Source: three-view drawing plus pictorial views. Frame: mm from the lowest corner of the part. A direction names the side the tool comes from. Coordinates: 2 decimals unless noted, no trailing zeros. Order: outer loops, then holes, each group sorted by start corner. A loop starts at its lowest first (then second) coordinate and runs counter-clockwise, first axis right, second up. Notation, with made-up numbers: (-27, 2) -> (8, 2) arc R10 ccw to (8, 16) -> close; hole circle Ø1 at (23, 0.25). An arc over 180 degrees is marked (long way). Use one line per item in the form item = value. Start each with the question number.
1) Ray query, line 1 along Y through (x, z) = (3.25, 24) (1 decimal); line 2 along Y through (x, z) = (11.25, 14.5) (1 decimal); line 3 along Y through (x, z) = (2.5, 11) (1 decimal). Return the intervals inside material, ascending.
2) Section query D-D on z = 31. Output: boundary loops of the cut face in (x, y) (1 decimal).
3) Section query B-B on z = 23.5. Output: boundary loops of the cut face in (x, y) (1 decimal).
4) Section query A-A on z = 10. Output: boundary loops of the cut face in (x, y) (1 decimal), then the cut area to 3 significant figures.
5) Access query for the marked faces 1, 2 and 3. Directions: +Z, -Z, +X, -X, +Y, -Y. A direction counts if a zero-diameter tool reaches every point of the face in a straight line with its end or side. Return the directions, or none.
6) Pin query (flat end, axial travel): pin 1 (3 mm diameter, centred on x = 6.92, y = 41.21, fed in from -Z); pin 2 (7 mm diameter, centred on x = 7, z = 30.5, fed in from -Y); pin 3 (8 mm diameter, centred on x = 6.92, y = 6.92, fed in from +Z) (1 decimal); pin 4 (2.5 mm diameter, centred on x = 6.5, y = 113, fed in from -Z). Return the tip coordinate at first contact, or that it passes through.
7) Section query C-C on y = 60. Output: boundary loops of the cut face in (x, z).
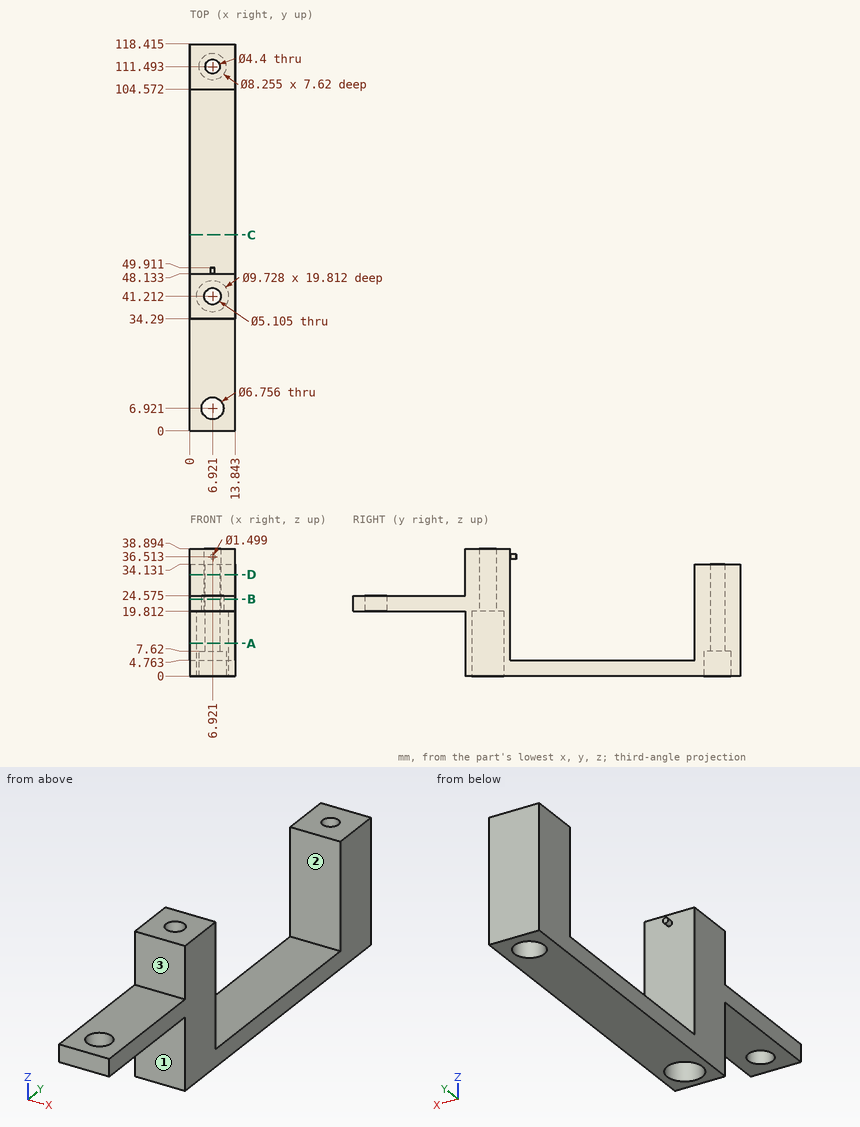
Answers below:
q1.line_1 = 0 to 48.1, 104.6 to 118.4
q1.line_2 = 34.3 to 39, 43.4 to 48.1, 104.6 to 118.4
q1.line_3 = 34.3 to 39.2, 43.2 to 48.1, 104.6 to 118.4
q2.outline = (0, 34.3) -> (13.8, 34.3) -> (13.8, 48.1) -> (0, 48.1) -> close; (0, 104.6) -> (13.8, 104.6) -> (13.8, 118.4) -> (0, 118.4) -> close; hole circle Ø5.1 at (6.9, 41.2); hole circle Ø4.4 at (6.9, 111.5)
q3.outline = (0, 0) -> (13.8, 0) -> (13.8, 48.1) -> (0, 48.1) -> close; (0, 104.6) -> (13.8, 104.6) -> (13.8, 118.4) -> (0, 118.4) -> close; hole circle Ø6.8 at (6.9, 6.9); hole circle Ø5.1 at (6.9, 41.2); hole circle Ø4.4 at (6.9, 111.5)
q4.outline = (0, 34.3) -> (13.8, 34.3) -> (13.8, 48.1) -> (0, 48.1) -> close; (0, 104.6) -> (13.8, 104.6) -> (13.8, 118.4) -> (0, 118.4) -> close; hole circle Ø9.7 at (6.9, 41.2); hole circle Ø4.4 at (6.9, 111.5)
q4.area = 294 mm^2
q5.face_1 = -Z, +X, -X, -Y
q5.face_2 = +Z, +X, -X
q5.face_3 = +Z, +X, -X, -Y
q6.pin_1 = through
q6.pin_2 = 34.29
q6.pin_3 = 24.6
q6.pin_4 = 7.62
q7.outline = (0, 0) -> (13.84, 0) -> (13.84, 4.76) -> (0, 4.76) -> close
